Read the model definition and answer for the solid it produces. Units are mm, in the model's axes. A direction names the side the tool comes from. Give positions to 0.01 mm unless a question says otherwise; leave off trailing zeros. Write each loop counter-clockwise with the first axis right and the second up, starting at its lowest first coordinate (ties: lowest second). Pieces come first, ordered by that corner, then holes. Notation, with made-up numbers: M 71.25,-17.5 L 129.25,-17.5 A7 cw 129.25,-11.5 Z; hole C -22,-25 d6. An arc over 180 degrees is marked long. Use a Markdown table: item, result. Add a question column.
Item 1: A cutting plane is placed at D-D on z = 11.5. Determine the outline of the cut face in (x, y).
Item 2: For faces 5 (the flat face through (0, 7, 0)), 6 (the flat face through (-11, 0, 2)), determine the directions among +Z, -Z, +X, -X, +Y, -Y from which every point of the face is accessible in a straight line to the end or side of a thin tool.
Item 3: A cutting plane is placed at A-A on x = -15. Determine the outline of the cut face in (y, z), then the cut area to 3 significant figures.
Item 4: A cutting plane is placed at C-C on y = 5. Determine the outline of the cut face in (x, z), then the cut area to 3 significant figures.
Item 5: The mould has two halves that part along X. Classify faces 1 (the cylindrical face through (-14.912, 0.098, 13.353)), 2 (the flat face through (0, 0, -17.25)), 3 (the flat face through (19, 0, 2)), 4 (the flat face through (25, 0, 0)): pulls with the +X half, pulls with the -X half, needs draft (parallel to the pull), parting line crosses it, or undercut.
Item 6: A cutting plane is placed at B-B on z = -2. Determine the outline of the cut face in (x, y), then the cut area to 3 significant figures.
Item 7: Consider probe 1 along X at (y, z) = (5.25, 9); probe 2 along Z at (x, y) = (-15, 3.25); probe 3 along X at (y, z) = (6, 11.5). Determine where each line is inside the solid, lowest interval first. Write a range as [from, to].
from build123d import *

# Parameters (mm, degrees)
SKETCH1_W           = 50
SKETCH1_H           = 34.5
BOSS_EXTRUDE1_DEPTH = 7


with BuildPart() as part:
    # Sketch1 → Boss-Extrude1 (new, symmetric)
    with BuildSketch(Plane(origin=(0, 0, 0), x_dir=(1, 0, 0), z_dir=(0, 1, 0))):
        Rectangle(SKETCH1_W, SKETCH1_H)
        with BuildLine():
            Line((-11, 5.646273024), (-11, -9.353726976))
            ThreePointArc((-11, -9.353726976), (-15, -13.353726976), (-19, -9.353726976))
            Line((-19, -9.353726976), (-19, 5.646273024))
            ThreePointArc((-19, 5.646273024), (-15, 9.646273024), (-11, 5.646273024))
        make_face(mode=Mode.SUBTRACT)
        with BuildLine():
            Line((11, 5.646273024), (11, -9.353726976))
            ThreePointArc((11, -9.353726976), (15, -13.353726976), (19, -9.353726976))
            Line((19, -9.353726976), (19, 5.646273024))
            ThreePointArc((19, 5.646273024), (15, 9.646273024), (11, 5.646273024))
        make_face(mode=Mode.SUBTRACT)
    extrude(amount=BOSS_EXTRUDE1_DEPTH, both=True)


solid = part.part
Filled in:
| question | item | result |
|---|---|---|
| 1 | outline | M -25,-7 L -18.38,-7 L -18.38,7 L -25,7 Z; M -11.62,-7 L 11.62,-7 L 11.62,7 L -11.62,7 Z; M 18.38,-7 L 25,-7 L 25,7 L 18.38,7 Z |
| 2 | face 5 | +Z, -Z, +X, -X, +Y |
| 2 | face 6 | +Y, -Y |
| 3 | outline | M -7,-17.25 L 7,-17.25 L 7,-9.65 L -7,-9.65 Z; M -7,13.35 L 7,13.35 L 7,17.25 L -7,17.25 Z |
| 3 | area | 161 mm² |
| 4 | outline | M -25,-17.25 L 25,-17.25 L 25,17.25 L -25,17.25 Z; hole M -19,-5.65 A4 ccw -11,-5.65 L -11,9.35 A4 ccw -19,9.35 Z; hole M 11,-5.65 A4 ccw 19,-5.65 L 19,9.35 A4 ccw 11,9.35 Z |
| 4 | area | 1,380 mm² |
| 5 | face 1 | undercut |
| 5 | face 2 | needs draft |
| 5 | face 3 | undercut |
| 5 | face 4 | pulls with the +X half |
| 6 | outline | M -25,-7 L -19,-7 L -19,7 L -25,7 Z; M -11,-7 L 11,-7 L 11,7 L -11,7 Z; M 19,-7 L 25,-7 L 25,7 L 19,7 Z |
| 6 | area | 476 mm² |
| 7 | probe 1 | [-25, -19], [-11, 11], [19, 25] |
| 7 | probe 2 | [-17.25, -9.65], [13.35, 17.25] |
| 7 | probe 3 | [-25, -18.38], [-11.62, 11.62], [18.38, 25] |
